Read the model definition and answer for the solid it produces. Units are mm, in the model's axes. A direction names the side the tool comes from. Coordinates: 2 decimals unless noted, no trailing zeros. Loops run counter-clockwise (first coordinate to the right, second up) from the corner with the lowest first, then second, coordinate; pieces in that order, holes last. Notation, with made-up numbers: M 28,77 L 60,77 A29 cw 60,116 Z; hole C -6.5,27.5 d5. An arc over 180 degrees is marked long. One line per item, written item: value. Start each with the question number.
1. The part is cut by section D-D (z = 10.5). Write down the section's boundary in (x, y) (1 decimal).
2. Consider probe 1 along Y at (x, z) = (0, 12.5) (1 decimal); probe 2 along Y at (x, z) = (0, 33) (3 decimals); probe 3 along Z at (x, y) = (1.5, -2.5). Determine where each line is inside the solid, lowest interval first.
3. For faces 1 (the face through (-0.107, -3.008, 9.392)), 2 (the face through (-2, 4, 44.45)), 3 (the face through (-0.881, -3.967, 35.058)), determine the directions among +Z, -Z, +X, -X, +Y, -Y from which every point of the face is accessible in a straight line to the end or side of a thin tool.
4. The part is cut by section B-B (y = 0). Write down the section's boundary in (x, z) (3 decimals).
5. The part is cut by section C-C (z = 33.5). Write down the section's boundary in (x, y) (3 decimals).
6. Flat-ended cylindrical pins translate along their axes: pin 1 (4.5 mm diameter, centred on x = 0, y = -0.5, fed in from -Z); pin 2 (4 mm diameter, centred on x = -3, z = 17, fed in from -Y); pin 3 (6 mm diameter, centred on y = -3, z = 7, fed in from -X) (3 decimals); pin 4 (2.5 mm diameter, centred on x = 0.5, y = 1.5, fed in from +Z). Find the tip coordinate at first contact, or state that the pin passes through.
7. Determine the mould class of faces 4 (the face through (0, 0, 25.4)), 5 (the face through (4.535, 3.477, 21.914)), 6 (the face through (-2.5, 2.5, 0)) for opening direction X: +X half, -X half, draft (parallel to the pull), parting line (faces both ways), or undercut.
```python
from build123d import *

# Parameters (mm, degrees)
SKETCH2_R           = 5.715
BOSS_EXTRUDE1_DEPTH = 19.05
CUT_EXTRUDE1_DEPTH  = 21.693596836
SKETCH9_R           = 5.715
BOSS_EXTRUDE5_DEPTH = 12.7
SKETCH10_R          = 5.715
BOSS_EXTRUDE6_DEPTH = 12.7
SKETCH11_R          = 4.064
CUT_EXTRUDE2_DEPTH  = 19.05


with BuildPart() as part:
    # Sketch2 → Boss-Extrude1 (new body)
    with BuildSketch(Plane.XY):
        with Locations(Location((0, 0, 0), (0, 0, 180))):
            Circle(SKETCH2_R)
    extrude(amount=BOSS_EXTRUDE1_DEPTH)

    # Sketch3 → Cut-Extrude1 (cut, through all)
    with BuildSketch(Plane(origin=(0, 0, 0), x_dir=(-1, 0, 0), z_dir=(0, 0, -1))):
        with BuildLine():
            Line((-1.710685757, 2.4765), (1.710685757, 2.4765))
            ThreePointArc((1.710685757, 2.4765), (0, -3.0099), (-1.710685757, 2.4765))
        make_face()
    extrude(amount=-CUT_EXTRUDE1_DEPTH, mode=Mode.SUBTRACT)

    # Sketch9 → Boss-Extrude5 (add)
    with BuildSketch(Plane.XY.offset(19.05)):
        with Locations(Location((0, 0, 0), (0, 0, 180))):
            Circle(SKETCH9_R)
    extrude(amount=BOSS_EXTRUDE5_DEPTH)

    # Sketch10 → Boss-Extrude6 (add)
    with BuildSketch(Plane.XY.offset(31.75)):
        with Locations(Location((0, 0, 0), (0, 0, 180))):
            Circle(SKETCH10_R)
    extrude(amount=BOSS_EXTRUDE6_DEPTH)

    # Sketch11 → Cut-Extrude2 (cut)
    with BuildSketch(Plane.XY.offset(44.45)):
        Circle(SKETCH11_R)
    extrude(amount=-CUT_EXTRUDE2_DEPTH, mode=Mode.SUBTRACT)


solid = part.part
```
Answer block:
1. outline: C 0,0 d11.4; hole M -1.7,2.5 A3 ccw long 1.7,2.5 Z
2. probe 1: y = -5.7 to -3, 2.5 to 5.7
2. probe 2: y = -5.715 to -4.064, 4.064 to 5.715
2. probe 3: z = 19.05 to 25.4
3. face 1: -Z
3. face 2: +Z, +X, -X, +Y, -Y
3. face 3: +Z
4. outline: M -5.715,0 L -3.01,0 L -3.01,19.05 L 3.01,19.05 L 3.01,0 L 5.715,0 L 5.715,44.45 L 4.064,44.45 L 4.064,25.4 L -4.064,25.4 L -4.064,44.45 L -5.715,44.45 Z
5. outline: C 0,0 d11.43; hole C 0,0 d8.128
6. pin 1: stops at z = 19.05
6. pin 2: stops at y = -5.63
6. pin 3: stops at x = -5.715
6. pin 4: stops at z = 25.4
7. face 4: undercut
7. face 5: parting line
7. face 6: draft
